```python
from build123d import *

# Parameters (mm, degrees)
F0_W         = 59.25
F0_H         = 1.5
F0_W_2       = 1.5
F0_H_2       = 59.25
F1_DEPTH     = 2
F0_W_3       = 140
F0_H_3       = 140
F2_DEPTH     = 32
F3_D         = 3
F4_R         = 5
F5_T1_DEPTH  = 49.25
F5_T3_DEPTH  = 49.25
F5_T5_DEPTH  = 49.25
F5_T7_DEPTH  = 49.25
F5_T12_ANGLE = 127.5884718038
F5_T15_ANGLE = 90
F5_T19_ANGLE = 127.5884718038
F5_T24_ANGLE = 127.5884718038
F5_T27_ANGLE = 90
F5_T31_ANGLE = 127.5884718038
F5_T36_ANGLE = 127.5884718038
F5_T39_ANGLE = 90
F5_T43_ANGLE = 127.5884718038
F5_T48_ANGLE = 127.5884718038
F5_T53_ANGLE = 127.5884718038
F5_T56_ANGLE = 90


# Not quite as in the source:
# - a fillet or chamfer that OpenCascade refuses, or shapes differently, is made with other operations: its cross-section is extruded or revolved along the edge and cut away or added


with BuildPart() as f1:
    # F0 (on Top) → F1 (new body)
    with BuildSketch(Plane.XY):
        with Locations((-36.375, 0)):
            Rectangle(F0_W, F0_H)
        with Locations((-6, 30.375)):
            Rectangle(F0_W_2, F0_H_2)
        with Locations((-6, -30.375)):
            Rectangle(F0_W_2, F0_H_2)
        with Locations((24.375, 0)):
            Rectangle(F0_W, F0_H)
        with Locations((-6, 0)):
            Rectangle(F0_W_2, F0_H)
    extrude(amount=F1_DEPTH)



with BuildPart() as f1b:
    # F0 (on Top) → F1, piece 2 (new body)
    with BuildSketch(Plane.XY):
        with Locations((-6, 0)):
            Rectangle(F0_W_3, F0_H_3)
        Polygon((55.5000009226, -35.6213207257), (29.6213207257, -61.5000009226), (-41.6213207257, -61.5000009226), (-67.5000009226, -35.6213207257), (-67.5000009226, 35.6213207257), (-41.6213207257, 61.5000009226), (29.6213207257, 61.5000009226), (55.5000009226, 35.6213207257), align=None, mode=Mode.SUBTRACT)
    extrude(amount=F1_DEPTH)


with BuildPart() as f1_1:
    add(f1.part)

    add(f1b.part)  # F2 merges F1b
    # F0 (on Top) → F2 (join)
    with BuildSketch(Plane.XY):
        Polygon((-41.6213207257, -61.5000009226), (29.6213207257, -61.5000009226), (55.5000009226, -35.6213207257), (55.5000009226, 35.6213207257), (29.6213207257, 61.5000009226), (-41.6213207257, 61.5000009226), (-67.5000009226, 35.6213207257), (-67.5000009226, -35.6213207257), align=None)
        Polygon((29, 60), (54, 35), (54, 0.75), (54, -0.75), (54, -35), (29, -60), (-5.25, -60), (-6.75, -60), (-41, -60), (-66, -35), (-66, -0.75), (-66, 0.75), (-66, 35), (-41, 60), (-6.75, 60), (-5.25, 60), align=None, mode=Mode.SUBTRACT)
    extrude(amount=F2_DEPTH)

    # F3 (through all)
    with Locations(Plane(origin=(0, 0, 0), x_dir=(1, 0, 0), z_dir=(0, 0, -1))):
        with Locations((-58.5, -52.5), (-58.5, 52.5), (46.5, 52.5), (46.5, -52.5)):
            Hole(F3_D / 2)

    # F4
    f4_edges = [f1_1.edges().sort_by_distance(p)[0] for p in [
        (-6.75, 60, 1),
        (-6.75, 0.75, 1),
        (-41, 60, 16),
        (-66, 35, 16),
        (-66, -0.75, 1),
        (-66, 0.75, 1),
        (-66, -35, 16),
        (-6.75, -0.75, 1),
        (-6.75, -60, 1),
        (29, -60, 16),
        (54, -35, 16),
        (54, -0.75, 1),
        (-5.25, -0.75, 1),
        (-5.25, -60, 1),
        (29, 60, 16),
        (54, 35, 16),
        (54, 0.75, 1),
        (-5.25, 0.75, 1),
        (-5.25, 60, 1),
        (-41, -60, 16),
        (-76, -70, 1),
        (64, -70, 1),
        (64, 70, 1),
        (-76, 70, 1),
        (-67.500001, -35.621321, 17),
        (-41.621321, -61.500001, 17),
        (29.621321, -61.500001, 17),
        (55.500001, -35.621321, 17),
        (55.500001, 35.621321, 17),
        (29.621321, 61.500001, 17),
        (-41.621321, 61.500001, 17),
        (-67.500001, 35.621321, 17),
    ]]
    fillet(f4_edges, radius=F4_R)

    # F5: chamfer of 0.75 on 20 edges, made by hand

    # F5_s2 → F5_t1 (cut)
    with BuildSketch(Plane.YZ.offset(-61)):
        Polygon((-0.75, 1.25), (0, 2), (-0.75, 2), align=None)
        Polygon((0.75, 1.25), (0, 2), (0.75, 2), align=None)
    extrude(amount=F5_T1_DEPTH, mode=Mode.SUBTRACT)

    # F5_s4 → F5_t3 (cut)
    with BuildSketch(Plane.YZ.offset(-0.25)):
        Polygon((-0.75, 1.25), (0, 2), (-0.75, 2), align=None)
        Polygon((0.75, 1.25), (0, 2), (0.75, 2), align=None)
    extrude(amount=F5_T3_DEPTH, mode=Mode.SUBTRACT)

    # F5_s6 → F5_t5 (cut)
    with BuildSketch(Plane.XZ.offset(-55)):
        Polygon((-5.25, 1.25), (-6, 2), (-5.25, 2), align=None)
        Polygon((-6.75, 1.25), (-6, 2), (-6.75, 2), align=None)
    extrude(amount=F5_T5_DEPTH, mode=Mode.SUBTRACT)

    # F5_s8 → F5_t7 (cut)
    with BuildSketch(Plane.XZ.offset(5.75)):
        Polygon((-6.75, 1.25), (-6, 2), (-6.75, 2), align=None)
        Polygon((-5.25, 1.25), (-6, 2), (-5.25, 2), align=None)
    extrude(amount=F5_T7_DEPTH, mode=Mode.SUBTRACT)


with BuildPart() as f5_tool10:
    # F5_s11 → F5_t12 (revolve)
    with BuildSketch(Plane(origin=(-19.9177172188, 25.8744507102, 0), x_dir=(0, 0, 1), z_dir=(0.6099857389, -0.7924123916, 0))):
        Polygon((1.25, 56.8445738842), (2, 57.5945738842), (2, 56.8445738842), align=None)
    revolve(axis=Axis((-61, -5.75, 2), (0, 0, -1)), revolution_arc=F5_T12_ANGLE)

    split(bisect_by=Plane.YZ.offset(-66), keep=Keep.TOP)


with BuildPart() as f1_2:
    add(f1_1.part)

    # F5_t9: cut F5_tool10
    add(f5_tool10.part, mode=Mode.SUBTRACT)

    # F5_s14 → F5_t15 (revolve, cut)
    with BuildSketch(Plane.YZ.offset(-11.75)):
        Polygon((-0.75, 1.25), (0, 2), (-0.75, 2), align=None)
    revolve(axis=Axis((-11.75, -5.75, 2), (0, 0, -1)), revolution_arc=F5_T15_ANGLE, mode=Mode.SUBTRACT)


with BuildPart() as f5_tool17:
    # F5_s18 → F5_t19 (revolve)
    with BuildSketch(Plane(origin=(19.2067847712, -14.7850600594, 0), x_dir=(0, 0, 1), z_dir=(-0.7924123916, 0.6099857389, 0))):
        Polygon((1.25, -55.7500139684), (2, -56.5000139684), (2, -55.7500139684), align=None)
    revolve(axis=Axis((-11.75, -55, 2), (0, 0, 1)), revolution_arc=F5_T19_ANGLE)

    split(bisect_by=Plane.XZ.offset(60), keep=Keep.BOTTOM)


with BuildPart() as f1_3:
    add(f1_2.part)

    # F5_t16: cut F5_tool17
    add(f5_tool17.part, mode=Mode.SUBTRACT)


with BuildPart() as f5_tool22:
    # F5_s23 → F5_t24 (revolve)
    with BuildSketch(Plane(origin=(15.4527259985, 20.0741276118, 0), x_dir=(0, 0, 1), z_dir=(-0.6099857389, -0.7924123916, 0))):
        Polygon((1.25, -47.3356251854), (2, -48.0856251854), (2, -47.3356251854), align=None)
    revolve(axis=Axis((49, -5.75, 2), (0, 0, 1)), revolution_arc=F5_T24_ANGLE)

    split(bisect_by=Plane.YZ.offset(54), keep=Keep.BOTTOM)


with BuildPart() as f1_4:
    add(f1_3.part)

    # F5_t21: cut F5_tool22
    add(f5_tool22.part, mode=Mode.SUBTRACT)

    # F5_s26 → F5_t27 (revolve, cut)
    with BuildSketch(Plane.YZ.offset(-0.25)):
        Polygon((-0.75, 1.25), (0, 2), (-0.75, 2), align=None)
    revolve(axis=Axis((-0.25, -5.75, 2), (0, 0, 1)), revolution_arc=F5_T27_ANGLE, mode=Mode.SUBTRACT)


with BuildPart() as f5_tool29:
    # F5_s30 → F5_t31 (revolve)
    with BuildSketch(Plane(origin=(-26.7417935508, -20.5853831579, 0), x_dir=(0, 0, 1), z_dir=(0.7924123916, 0.6099857389, 0))):
        Polygon((1.25, 48.4301851013), (2, 49.1801851013), (2, 48.4301851013), align=None)
    revolve(axis=Axis((-0.25, -55, 2), (0, 0, -1)), revolution_arc=F5_T31_ANGLE)

    split(bisect_by=Plane.XZ.offset(60), keep=Keep.BOTTOM)


with BuildPart() as f1_5:
    add(f1_4.part)

    # F5_t28: cut F5_tool29
    add(f5_tool29.part, mode=Mode.SUBTRACT)


with BuildPart() as f5_tool34:
    # F5_s35 → F5_t36 (revolve)
    with BuildSketch(Plane(origin=(19.2067847712, 14.7850600594, 0), x_dir=(0, 0, 1), z_dir=(-0.7924123916, -0.6099857389, 0))):
        Polygon((1.25, 55.7500139684), (2, 56.5000139684), (2, 55.7500139684), align=None)
    revolve(axis=Axis((-11.75, 55, 2), (0, 0, -1)), revolution_arc=F5_T36_ANGLE)

    split(bisect_by=Plane.XZ.offset(-60), keep=Keep.TOP)


with BuildPart() as f1_6:
    add(f1_5.part)

    # F5_t33: cut F5_tool34
    add(f5_tool34.part, mode=Mode.SUBTRACT)

    # F5_s38 → F5_t39 (revolve, cut)
    with BuildSketch(Plane.XZ.offset(-5.75)):
        Polygon((-6.75, 1.25), (-6, 2), (-6.75, 2), align=None)
    revolve(axis=Axis((-11.75, 5.75, 2), (0, 0, -1)), revolution_arc=F5_T39_ANGLE, mode=Mode.SUBTRACT)


with BuildPart() as f5_tool41:
    # F5_s42 → F5_t43 (revolve)
    with BuildSketch(Plane(origin=(-19.9177172188, -25.8744507102, 0), x_dir=(0, 0, 1), z_dir=(0.6099857389, 0.7924123916, 0))):
        Polygon((1.25, -56.8445738842), (2, -57.5945738842), (2, -56.8445738842), align=None)
    revolve(axis=Axis((-61, 5.75, 2), (0, 0, 1)), revolution_arc=F5_T43_ANGLE)

    split(bisect_by=Plane.YZ.offset(-66), keep=Keep.TOP)


with BuildPart() as f1_7:
    add(f1_6.part)

    # F5_t40: cut F5_tool41
    add(f5_tool41.part, mode=Mode.SUBTRACT)


with BuildPart() as f5_tool46:
    # F5_s47 → F5_t48 (revolve)
    with BuildSketch(Plane(origin=(-26.7417935508, 20.5853831579, 0), x_dir=(0, 0, 1), z_dir=(0.7924123916, -0.6099857389, 0))):
        Polygon((1.25, -48.4301851013), (2, -49.1801851013), (2, -48.4301851013), align=None)
    revolve(axis=Axis((-0.25, 55, 2), (0, 0, 1)), revolution_arc=F5_T48_ANGLE)

    split(bisect_by=Plane.XZ.offset(-60), keep=Keep.TOP)


with BuildPart() as f1_8:
    add(f1_7.part)

    # F5_t45: cut F5_tool46
    add(f5_tool46.part, mode=Mode.SUBTRACT)


with BuildPart() as f5_tool51:
    # F5_s52 → F5_t53 (revolve)
    with BuildSketch(Plane(origin=(15.4527259985, -20.0741276118, 0), x_dir=(0, 0, 1), z_dir=(-0.6099857389, 0.7924123916, 0))):
        Polygon((1.25, 47.3356251854), (2, 48.0856251854), (2, 47.3356251854), align=None)
    revolve(axis=Axis((49, 5.75, 2), (0, 0, -1)), revolution_arc=F5_T53_ANGLE)

    split(bisect_by=Plane.YZ.offset(54), keep=Keep.BOTTOM)


with BuildPart() as f1_9:
    add(f1_8.part)

    # F5_t50: cut F5_tool51
    add(f5_tool51.part, mode=Mode.SUBTRACT)

    # F5_s55 → F5_t56 (revolve, cut)
    with BuildSketch(Plane.XZ.offset(-5.75)):
        Polygon((-5.25, 1.25), (-6, 2), (-5.25, 2), align=None)
    revolve(axis=Axis((-0.25, 5.75, 2), (0, 0, 1)), revolution_arc=F5_T56_ANGLE, mode=Mode.SUBTRACT)


solid = f1_9.part
```
Verification items for the finished model (mm, model axes). A direction names the side the tool comes from. Give positions to 0.01 mm unless a question says otherwise; leave off trailing zeros. Order: outer loops, then holes, each group sorted by start corner. A loop starts at its lowest first (then second) coordinate and runs counter-clockwise, first axis right, second up. Notation, with made-up numbers: (27, -7.5) -> (52, -7.5) arc R13 cw to (52, 13.5) -> close; hole circle Ø3 at (-37, 37). An arc over 180 degrees is marked (long way). Use a Markdown table: item, result.
1) Depth check by flat-ended pin: pin 1 Ø6 at (x, z) = (-12.5, 21.5) entering from +Y; pin 2 Ø6 at (y, z) = (-2, 15) entering from +X; pin 3 Ø2.5 at (x, y) = (-58.5, -52.5) entering from -Z; pin 4 Ø12 at (y, z) = (34, 8.5) entering from -X. Enter the tip coordinate at first touch or a pass-through.
Results:
| item | result |
|---|---|
| pin 1 | y = 61.5 |
| pin 2 | x = 55.5 |
| pin 3 | through |
| pin 4 | x = -67.5 |
2) Material ranges on probe 1 along X at (y, z) = (-8.5, 22); probe 2 along X at (y, z) = (-52.5, 0.85); probe 3 along Y at (x, z) = (-21.5, 5), recorded low to high.
Results:
| item | result |
|---|---|
| probe 1 | -67.5 to -66, 54 to 55.5 |
| probe 2 | -76 to -60, -57 to -48.5, -6.75 to -5.25, 36.5 to 45, 48 to 64 |
| probe 3 | -61.5 to -60, 60 to 61.5 |
3) Tool access check on faces 5 (the cylindrical face through (-75, -68, 1)), 6 (the flat face through (-54.72, -48.4, 16.79)), 7 (the cylindrical face through (29.49, 61.11, 17.21)), 8 (the cylindrical face through (-64.57, 2.25, 0.63)), 9 (the conical face through (-64.037, 1.512, 1.464)). Record the directions out of +Z, -Z, +X, -X, +Y, -Y that give a thin tool (end or side, any length) a straight path to the whole face; none if there is none.
Results:
| item | result |
|---|---|
| face 5 | +Z, -Z, -X, -Y |
| face 6 | +Z, -X, -Y |
| face 7 | +Z, +X, +Y |
| face 8 | +Z, -Z |
| face 9 | +Z |
4) Section check A-A, the plane y = 24. Record the boundary of the cut face in (x, z).
Results:
| item | result |
|---|---|
| outline | (-76, 0) -> (-66, 0) -> (-66, 32) -> (-67.5, 32) -> (-67.5, 2) -> (-76, 2) -> close; (-6.75, 0) -> (-5.25, 0) -> (-5.25, 1.25) -> (-6, 2) -> (-6.75, 1.25) -> close; (54, 0) -> (64, 0) -> (64, 2) -> (55.5, 2) -> (55.5, 32) -> (54, 32) -> close |
5) Mould release check, pull along X, two halves, no side actions. Record for faces 1 (the cylindrical face through (-8.18, 2.25, 0.63)), 2 (the flat face through (-6, 61.5, 17)), 3 (the cylindrical face through (-41.44, -61.13, 17.21)), 4 (the flat face through (-65, 0, 2)): pulls with the +X half, pulls with the -X half, needs draft (parallel to the pull), parting line crosses it, or undercut.
Results:
| item | result |
|---|---|
| face 1 | undercut |
| face 2 | needs draft |
| face 3 | pulls with the -X half |
| face 4 | undercut |
6) Section check C-C, the plane y = -40. Record the boundary of the cut face in (x, z).
Results:
| item | result |
|---|---|
| outline | (-76, 0) -> (-61, 0) -> (-61, 32) -> (-63.12, 32) -> (-63.12, 2) -> (-76, 2) -> close; (-6.75, 0) -> (-5.25, 0) -> (-5.25, 1.25) -> (-6, 2) -> (-6.75, 1.25) -> close; (49, 0) -> (64, 0) -> (64, 2) -> (51.12, 2) -> (51.12, 32) -> (49, 32) -> close |
